Here's the drawing with two shaded views (mm, measured from the low corner). I have some questions. Round coordinates to 2 decimals unless told otherwise and drop trailing zeros. Loops run counter-clockwise (first coordinate to the right, second up) from the corner with the lowest first, then second, coordinate; pieces in that order, holes last. Notation, with made-up numbers: M 72,66.5 L 117,66.5 A11 cw 117,78.5 Z; hole C 32.5,-1 d1. An arc over 180 degrees is marked long. Write each question's results on one line, items separated by ' | '. Start each with the question number.
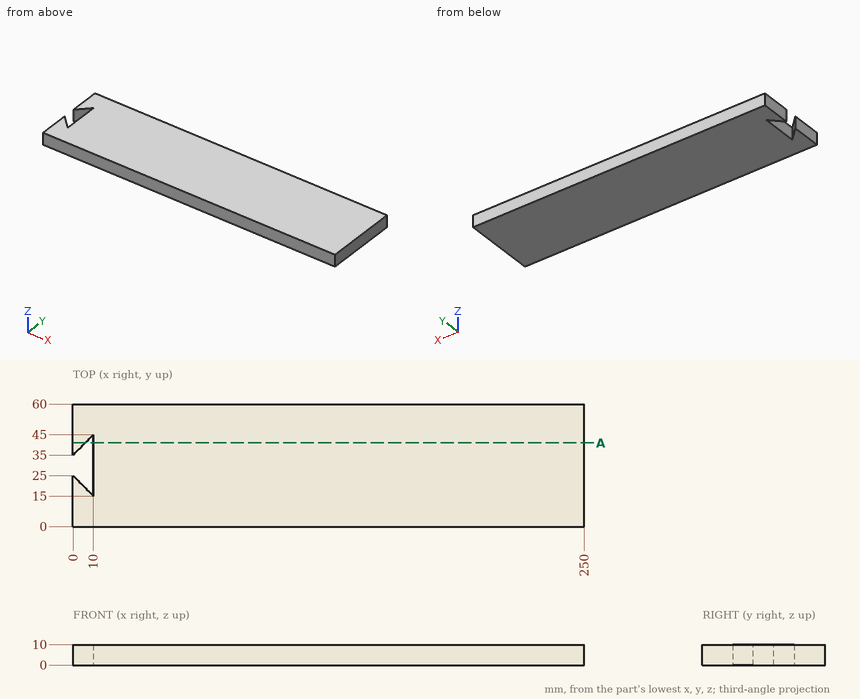
Item 1: I need wall thicknesses on L1, parallel to X at y = 32, z = 7.5; L2, parallel to X at y = 24, z = 7.5; L3, parallel to X at y = 43.5, z = 5.75. Which ranges of each line are inside material? Lowest first, please.
Item 2: I'm going to push flat-ended pins straight in: pin 1 (8 mm diameter, centred on x = 70.5, y = 21.5, fed in from -Z); pin 2 (3 mm diameter, centred on y = 29, z = 4.5, fed in from -X). Where does each tip first touch, or does it pass through?
Item 3: If we section it at A-A on y = 41: Please give me the cut outline in (x, z).
Numbers:
1) L1: 10 to 250 | L2: 0 to 1, 10 to 250 | L3: 0 to 8.5, 10 to 250
2) pin 1: z = 0 | pin 2: x = 10
3) outline: M 0,0 L 6,0 L 6,10 L 0,10 Z; M 10,0 L 250,0 L 250,10 L 10,10 Z
